from build123d import *

# Parameters (mm, degrees)
CUT_EXTRUDE1_DEPTH      = 21.101424287
CUT_EXTRUDE1_DEPTH_BACK = 21.101424287
CUT_EXTRUDE2_DEPTH      = 21.101424287
CUT_EXTRUDE2_DEPTH_BACK = 21.101424287
FILLET2_R               = 0.254
CUT_EXTRUDE3_DEPTH      = 21.101424287
CUT_EXTRUDE3_DEPTH_BACK = 21.101424287
SKETCH7_W               = 2.38125
SKETCH7_H               = 17.740225881


with BuildPart() as part:
    # Sketch2 → Revolve1 (revolve)
    with BuildSketch(Plane(origin=(0, 0, 0), x_dir=(0, 0, -1), z_dir=(1, 0, 0)), mode=Mode.PRIVATE) as revolve1_sk:
        with BuildLine():
            Line((-18.8214, 0), (-18.8214, 1.190625))
            Line((-18.8214, 1.190625), (-2.0574, 1.190625))
            ThreePointArc((-2.0574, 1.190625), (-1.561820484, 3.310560517), (-0.1778, 4.9911))
            Line((-0.1778, 4.9911), (0, 4.9911))
            Line((0, 4.9911), (0, 2.38125))
            Line((0, 2.38125), (8.382, 2.38125))
            Line((8.382, 2.38125), (8.382, 2.24506403))
            Line((8.382, 2.24506403), (8.382, 0))
            Line((8.382, 0), (-18.8214, 0))
        make_face()
    revolve(revolve1_sk.sketch.rotate(Axis((0, 0, 18.8214), (0, 0, -1)), 90), axis=Axis((0, 0, 18.8214), (0, 0, -1)))

    # Sketch3 → Cut-Extrude1 (cut, two sides: drawn at the far end of the back side and taken through both)
    with BuildSketch(Plane(origin=(0, 0, 0), x_dir=(1, 0, 0), z_dir=(0, 1, 0)).offset(-CUT_EXTRUDE1_DEPTH_BACK)):
        Polygon((0, -18.8214), (1.393825, -17.004931895), (1.393825, -19.3294), (-1.393825, -19.3294), (-1.393825, -17.004931895), align=None)
    extrude(amount=CUT_EXTRUDE1_DEPTH + CUT_EXTRUDE1_DEPTH_BACK, mode=Mode.SUBTRACT)

    # Sketch5 → Cut-Extrude2 (cut, two sides: drawn at the far end of the back side and taken through both)
    with BuildSketch(Plane(origin=(0, 0, 0), x_dir=(0, 0, -1), z_dir=(1, 0, 0)).offset(-CUT_EXTRUDE2_DEPTH_BACK)):
        Polygon((-18.8214, 0), (-17.26974729, 1.508125), (-19.1389, 1.508125), (-19.1389, -1.508125), (-17.26974729, -1.508125), align=None)
    extrude(amount=CUT_EXTRUDE2_DEPTH + CUT_EXTRUDE2_DEPTH_BACK, mode=Mode.SUBTRACT)

    # Fillet2
    fillet2_edges = [part.edges().sort_by_distance(p)[0] for p in [
        (-2.38125, 0, 0),
    ]]
    fillet(fillet2_edges, radius=FILLET2_R)

    # Sketch7 → Cut-Extrude3 (cut, two sides: drawn at the far end of the back side and taken through both)
    with BuildSketch(Plane(origin=(0, 0, 0), x_dir=(1, 0, 0), z_dir=(0, 1, 0)).offset(-CUT_EXTRUDE3_DEPTH_BACK)):
        with Locations((0, -10.927512941)):
            Rectangle(SKETCH7_W, SKETCH7_H)
    extrude(amount=CUT_EXTRUDE3_DEPTH + CUT_EXTRUDE3_DEPTH_BACK, mode=Mode.SUBTRACT)


solid = part.part
Here's how the part is built. I have some questions about the finished solid (model axes, mm). A direction names the side the tool comes from. Give positions to 0.01 mm unless a question says otherwise; leave off trailing zeros. Write each loop counter-clockwise with the first axis right and the second up, starting at its lowest first coordinate (ties: lowest second). Pieces come first, ordered by that corner, then holes. Notation, with made-up numbers: (50.25, -2) -> (72.25, -2) arc R31 ccw to (72.25, 29) -> close; hole circle Ø7 at (-7, 39.5). An arc over 180 degrees is marked (long way). Use one line per item in the form item = value. Start each with the question number.
1. Will these pins go through, and if not, where does the flat tip stop? pin 1 Ø1 at (x, y) = (-2, 3) entering from -Z; pin 2 Ø3 at (x, z) = (2, -3) entering from -Y; pin 3 Ø2 at (y, z) = (-2.5, -5.5) entering from +X.
2. If I drill on L1, parallel to X at y = -0.5, z = -4.5; L2, parallel to Z at x = -3.5, y = -2.5; L3, parallel to X at y = -1.5, z = -6.75, over which ranges is the centre line in solid material (lowest first)?
3. On a 3-axis mill with a long thin cutter (end or side, diameter ignored), from which of +Z, -Z, +X, -X, +Y, -Y can I reach the whole of each face in a straight line? I mean faces 1 (the face through (0, 0, 2.057)), 2 (the face through (2, 2, 0)). Say none if no direction works.
4. Imagine slicing it at A-A on z = -6. List the corners of the cut face in (x, y) for me.
Entries:
q1.pin_1 = 0
q1.pin_2 = -2.33
q1.pin_3 = 1.85
q2.L1 = -2.33 to 2.33
q2.L2 = 0 to 0.91
q2.L3 = -1.85 to 1.85
q3.face_1 = +Z, +X, -X, +Y, -Y
q3.face_2 = -Z
q4.outline = circle Ø4.76 at (0, 0)
